For this review, use the dimensioned drawing (mm, ordinates from the lowest corner) and the shaded views. Round coordinates to 2 decimals unless told otherwise and drop trailing zeros. Write each loop counter-clockwise with the first axis right and the second up, starting at its lowest first coordinate (ties: lowest second). Pieces come first, ordered by that corner, then holes. Notation, with made-up numbers: M 5,-40 L 22,-40 A16 ccw 22,-33 Z; hole C 61,-16.5 d10. An arc over 180 degrees is marked long. Use one line per item in the form item = value. Start each with the question number.
Item 1: Add section D-D (z = 4.5). State the section outline as (x, y) points, and give its area (3 significant figures).
Item 2: Add section B-B (x = 19.5). State the section outline as (y, z) points.
Item 3: Add section A-A (z = 15.5). State the section outline as (x, y) points.
Item 4: Add section C-C (y = 4). State the section outline as (x, z) points.
Item 5: For P1, Ø1.6, axis at x = 29, z = 15.5, coming from the +Y side, flat-tipped, find the tip position at first contact; note if it passes through.
Item 6: Draft analysis for pull direction Z (two halves, no side actions). For the marked faces 1, 2, 3 and 4, state which applies: released by +Z, released by -Z, zero draft, split by the parting line, or undercut.
Item 7: For line 1 (X direction, y = 2.75, z = 15.5); line 2 (X direction, y = 5.5, z = 4.5); line 3 (X direction, y = 4, z = 18.5), list the stretches that pass through material, from the lowest coordinate up. Write a range as [from, to].
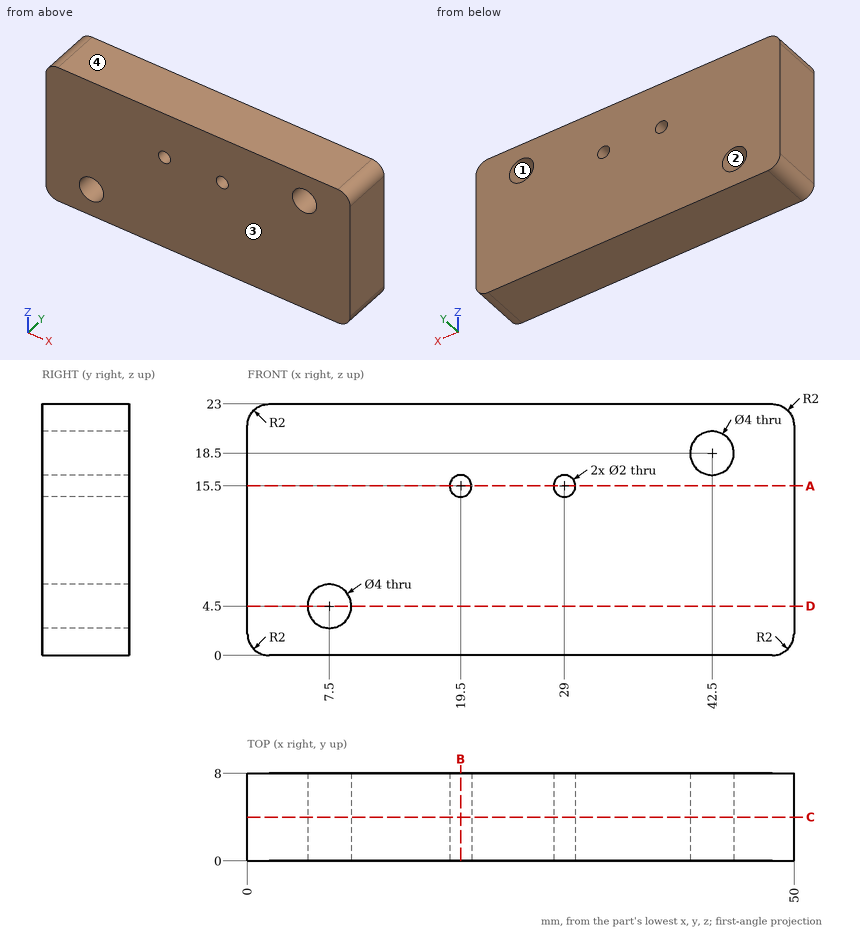
Calculated:
q1.outline = M 0,0 L 5.5,0 L 5.5,8 L 0,8 Z; M 9.5,0 L 50,0 L 50,8 L 9.5,8 Z
q1.area = 368 mm^2
q2.outline = M 0,0 L 8,0 L 8,14.5 L 0,14.5 Z; M 0,16.5 L 8,16.5 L 8,23 L 0,23 Z
q3.outline = M 0,0 L 18.5,0 L 18.5,8 L 0,8 Z; M 20.5,0 L 28,0 L 28,8 L 20.5,8 Z; M 30,0 L 50,0 L 50,8 L 30,8 Z
q4.outline = M 0,2 A2 ccw 2,0 L 48,0 A2 ccw 50,2 L 50,21 A2 ccw 48,23 L 2,23 A2 ccw 0,21 Z; hole C 7.5,4.5 d4; hole C 19.5,15.5 d2; hole C 29,15.5 d2; hole C 42.5,18.5 d4
q5.P1 = through
q6.face_1 = undercut
q6.face_2 = undercut
q6.face_3 = zero draft
q6.face_4 = released by +Z
q7.line_1 = [0, 18.5], [20.5, 28], [30, 50]
q7.line_2 = [0, 5.5], [9.5, 50]
q7.line_3 = [0, 40.5], [44.5, 50]
